Part model, mm, in its own coordinate system. Round coordinates to 2 decimals unless told otherwise and drop trailing zeros. Write each loop counter-clockwise with the first axis right and the second up, starting at its lowest first coordinate (ties: lowest second). Pieces come first, ordered by that corner, then holes. Notation, with made-up numbers: M 54.5,67 L 76.5,67 A21 ccw 76.5,105 Z; hole C 79.25,5.25 d3. An arc over 180 degrees is marked long. Answer as a JSON object with one key per item and string values. Group by question number.
1. Band-saw the part on C-C, the plane y = 3.2. Count the separate pieces of the cut face and the enclosed holes in it, plus the area to 3 significant figures.
2. Band-saw the part on D-D, the plane x = 17.5. Write the cut outline in (y, z), plus the area to 3 significant figures.
3. Drill centre lines: line 1 (X direction, y = 2.4, z = 0); line 2 (Z direction, x = 0, y = 2.85); line 3 (X direction, y = 0.25, z = 1). Where is each one in solid material? Low to high. Write a range as from..to.
4. Band-saw the part on A-A, the plane x = 26. Write the cut outline in (y, z).
5. Band-saw the part on B-B, the plane x = 0. Write the cut outline in (y, z).
6. Drop flat-ended pins along their axis: pin 1 (16 mm diameter, centred on x = 0, z = 0, fed in from +Y); pin 2 (1.5 mm diameter, centred on x = 1, y = 1.5, fed in from +Z). Give the stop position or say it passes through.
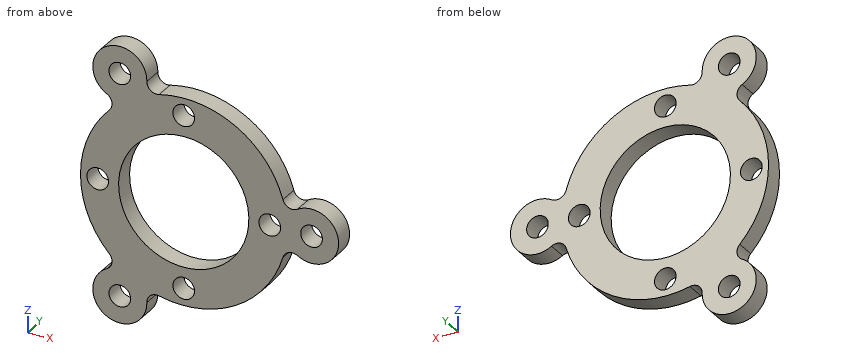
Autodesk Inventor part; units mm, degrees
ref_plane "YZ Plane" through (0, 0, 0) normal (1, 0, 0) x (0, 1, 0)
ref_plane "XZ Plane" through (0, 0, 0) normal (0, 1, 0) x (-1, 0, 0)
ref_plane "XY Plane" through (0, 0, 0) normal (0, 0, 1) x (1, 0, 0)
sketch "Sketch1" plane through (0, 0, 0) normal (0, 1, 0) x (-1, 0, 0)
  circle A0 centre (0, 0) radius 21
  dimension "d0" = 42
extrude "Extrusion1" add sketch "Sketch1" along normal blind 4
sketch "Sketch2" plane through (0, 4, 0) normal (0, 1, 0) x (1, 0, 0)
  circle A0 centre (0, 0) radius 21
hole "Hole1" at (0, 4, 0) direction (0, -1, 0) diameter 26.5 end through all
sketch "Sketch3" plane through (0, 4, 0) normal (0, 1, 0) x (1, 0, 0)
  circle A0 centre (26, 0) radius 2.2
  line L0 (26, 0) -> (0, 0) construction
  circle A1 centre (26, 0) radius 5.5
  circle A2 centre (0, 0) radius 21
  circle A3 centre (-13, 22.5167) radius 2.2
  circle A4 centre (-13, 22.5167) radius 5.5
  circle A5 centre (-13, -22.5167) radius 2.2
  circle A6 centre (-13, -22.5167) radius 5.5
  dimension "d10" = 4.4
  dimension "d11" = 11
  dimension "d14" = 360
  dimension "d19" = 26
extrude "Extrusion2" add sketch "Sketch3" against normal blind 4 contours A1 A2 | A2 A1 | A4 A2 | A2 A4 | A6 A2 | A2 A6
fillet "Fillet1" radius 2 6 edges at (20.899, 2, -2.0567) (20.899, 2, 2.0567) (-12.2307, 2, 17.0707) (-8.6683, 2, 19.1275) (-12.2307, 2, -17.0707) (-8.6683, 2, -19.1275)
sketch "Sketch4" plane through (0, 4, 0) normal (0, 1, 0) x (1, 0, 0)
  circle A0 centre (-17.5, 0) radius 2.2
  line L0 (-17.5, 0) -> (0, 0) construction
  circle A1 centre (0, -17.5) radius 2.2
  circle A2 centre (17.5, 0) radius 2.2
  circle A3 centre (0, 17.5) radius 2.2
  dimension "d20" = 4.4
  dimension "d22" = 17.5
  dimension "d25" = 360
extrude "Extrusion3" cut sketch "Sketch4" against normal blind 4
properties part number "775 Mounting plate" material "Aluminum 6061"
Worked answers:
{
 "1": {"separate pieces": "1", "enclosed holes": "8", "area": "1,020 mm^2"},
 "2": {"outline": "M 0,-11.61 L 4,-11.61 L 4,-2.2 L 0,-2.2 Z; M 0,2.2 L 4,2.2 L 4,11.61 L 0,11.61 Z", "area": "75.3 mm^2"},
 "3": {"line 1": "x = -21..-19.7, -15.3..-13.25, 13.25..15.3, 19.7..23.8, 28.2..31.5", "line 2": "z = -21..-19.7, -15.3..-13.25, 13.25..15.3, 19.7..21", "line 3": "x = -20.98..-19.46, -15.54..-13.21, 13.21..15.54, 19.46..24.04, 27.96..31.41"},
 "4": {"outline": "M 0,-5.5 L 4,-5.5 L 4,-2.2 L 0,-2.2 Z; M 0,2.2 L 4,2.2 L 4,5.5 L 0,5.5 Z"},
 "5": {"outline": "M 0,-21 L 4,-21 L 4,-19.7 L 0,-19.7 Z; M 0,-15.3 L 4,-15.3 L 4,-13.25 L 0,-13.25 Z; M 0,13.25 L 4,13.25 L 4,15.3 L 0,15.3 Z; M 0,19.7 L 4,19.7 L 4,21 L 0,21 Z"},
 "6": {"pin 1": "passes through", "pin 2": "stops at z = 21"}
}
